from build123d import *

# Parameters (mm, degrees)
THREAD1_PITCH = 0.8


with BuildPart() as part:
    # Sketch1 → Revolve1 (revolve)
    with BuildSketch(Plane(origin=(0, 0, 0), x_dir=(0, 0, -1), z_dir=(1, 0, 0))):
        Polygon((1778.036254975, 1559.979920793), (1775.536254975, 1565.487394057), (1775.536254975, 1568.979920793), (1776.536254975, 1568.979920793), (1780.036254975, 1559.979920793), (1780.036254975, 1554.979920793), (1778.036254975, 1554.979920793), align=None)
    revolve(axis=Axis((0, 1554.979920793, -1773.036254975), (0, 1, 0)))

    # Thread1: the profile of Thread Profile1 profile screwed along a right-hand helix of 4.375 turns, 8 arcs to a turn; built about Z, then put on its axis
    thread1_z = Axis((0, 0, 0), (0, 0, 1))
    thread1_corners = [(2.5003, 0, 0.600173208), (2.066987296, 0, 0.350000001), (2.066987296, 0, 0.250000001), (2.5003, 0, -0.000173205)]
    with BuildLine(mode=Mode.PRIVATE) as thread1_profile:
        Line(thread1_corners[0], thread1_corners[1])
        Line(thread1_corners[1], thread1_corners[2])
        Line(thread1_corners[2], thread1_corners[3])
        Line(thread1_corners[3], thread1_corners[0])
    thread1_cap = Face(thread1_profile.wire())
    thread1_turn_angles = [0, 22.5, 45, 67.5, 90, 112.5, 135, 157.5, 180, 202.5, 225, 247.5, 270, 292.5, 315, 337.5, 360]
    thread1_turn_weights = [1, 0.9238795325112867, 1, 0.9238795325112867, 1, 0.9238795325112867, 1, 0.9238795325112867, 1, 0.9238795325112867, 1, 0.9238795325112867, 1, 0.9238795325112867, 1, 0.9238795325112867, 1]
    thread1_turn_rails = [Edge.make_bspline([Vector(p[0], p[1], 0).rotate(thread1_z, thread1_turn_angles[k]) / thread1_turn_weights[k] + Vector(0, 0, p[2] + THREAD1_PITCH * thread1_turn_angles[k] / 360) for k in range(17)], [0, 0, 0, 1, 1, 2, 2, 3, 3, 4, 4, 5, 5, 6, 6, 7, 7, 8, 8, 8], 2, thread1_turn_weights) for p in thread1_corners]
    thread1_turn_sides = [Face.make_surface_from_curves(thread1_turn_rails[p[0]], thread1_turn_rails[p[1]]) for p in [(0, 1), (1, 2), (2, 3), (3, 0)]]
    thread1_last_angles = [1440, 1462.5, 1485, 1507.5, 1530, 1552.5, 1575]
    thread1_last_weights = [1, 0.9238795325112867, 1, 0.9238795325112867, 1, 0.9238795325112867, 1]
    thread1_last_rails = [Edge.make_bspline([Vector(p[0], p[1], 0).rotate(thread1_z, thread1_last_angles[k]) / thread1_last_weights[k] + Vector(0, 0, p[2] + THREAD1_PITCH * thread1_last_angles[k] / 360) for k in range(7)], [0, 0, 0, 1, 1, 2, 2, 3, 3, 3], 2, thread1_last_weights) for p in thread1_corners]
    thread1_last_sides = [Face.make_surface_from_curves(thread1_last_rails[p[0]], thread1_last_rails[p[1]]) for p in [(0, 1), (1, 2), (2, 3), (3, 0)]]
    thread1 = Plane(origin=(0, 1568.979920793, -1773.036254975), x_dir=(-1, 0, 0), z_dir=(0, -1, 0)) * Solid(Shell([*[p.moved(Location((0, 0, THREAD1_PITCH * i))) for i in range(4) for p in thread1_turn_sides], *thread1_last_sides, thread1_cap, thread1_cap.rotate(thread1_z, 1575).moved(Location((0, 0, THREAD1_PITCH * 1575 / 360)))]))
    add(thread1)


solid = part.part
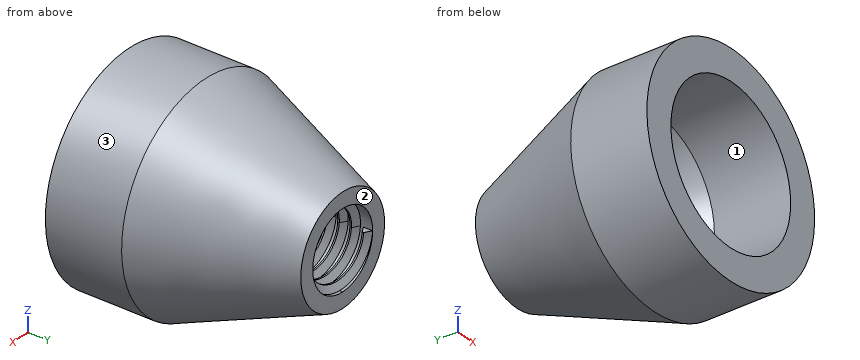
Source: CAD feature listing. Evaluate the final solid. Frame: model axes, mm. Face numbers are marked on the shaded views. Coordinates: 2 decimals unless noted, no trailing zeros. Order: outer loops, then holes, each group sorted by start corner. A loop starts at its lowest first (then second) coordinate and runs counter-clockwise, first axis right, second up. Notation, with made-up numbers: M -24.5,23 L -10.5,23 A21 cw -10.5,50 Z; hole C 7.25,23 d10. An arc over 180 degrees is marked long. Write each question's results on one line, items separated by ' | '. Start each with the question number.
Item 1: Draft query along X for the marked faces 1, 2 and 3. Return one class per face: pulls with the +X half, pulls with the -X half, needs draft (parallel to the pull), parting line crosses it, or undercut.
Item 2: Cut plane C-C (y = 1564.5). Return loops of the section in (x, z), and give its area (3 significant figures).
Item 3: Cut plane B-B (z = -1770.75). Count the separate pieces of the cut face and the enclosed holes in it, and give its area (3 significant figures).
Item 4: Cut plane A-A (y = 1556). Return loops of the section in (x, z), and give its area (3 significant figures).
Item 5: First-contact query: pin 1 Ø5 at (x, y) = (4, 1566) entering from -Z (3 decimals); pin 2 Ø5 at (x, y) = (0.5, 1567) entering from +Z; pin 3 Ø3 at (y, z) = (1567.5, -1774.5) entering from -X; pin 4 Ø3 at (x, z) = (0, -1773.04) entering from -Y. Flat tips, straight axial feed; report the tip coordinate or a pass-through.
Item 6: Line query: probe 1 along Y at (x, z) = (0.75, -1771); probe 2 along Z at (x, y) = (-4, 1559.5); probe 3 along Z at (x, y) = (0, 1566.35). Output: solid intervals per line, ascending.
Checked values:
1) face 1: undercut | face 2: needs draft | face 3: parting line crosses it
2) outline: C 0,-1773.04 d10.48; hole C 0,-1773.04 d5.9 | area: 59.0 mm2
3) separate pieces: 1 | enclosed holes: 3 | area: 70.7 mm2
4) outline: C 0,-1773.04 d14; hole C 0,-1773.04 d10 | area: 75.4 mm2
5) pin 1: stops at z = -1777.895 | pin 2: stops at z = -1767.8 | pin 3: stops at x = -4.53 | pin 4: passes through
6) probe 1: y = 1565.62 to 1565.83, 1566.42 to 1566.63, 1567.22 to 1567.43, 1568.02 to 1568.23 | probe 2: z = -1778.78 to -1776.04, -1770.04 to -1767.29 | probe 3: z = -1777.56 to -1775.48, -1770.83 to -1768.51
